from build123d import *

# Parameters (mm, degrees)
SKETCH1_R               = 32
BOSS_EXTRUDE1_DEPTH     = 15
SKETCH1_R_2             = 19
BOSS_EXTRUDE1_2_DEPTH   = 15
BOSS_EXTRUDE2_DEPTH     = 5
CUT_EXTRUDE1_DEPTH      = 84.026980949
CUT_EXTRUDE1_DEPTH_BACK = 84.026980949
SKETCH1_4_R             = 17
SKETCH1_4_R_2           = 10
BOSS_EXTRUDE3_START     = 15
SKETCH1_5_R             = 21.5
SKETCH1_5_R_2           = 17
BOSS_EXTRUDE3_DEPTH     = 15
CUT_EXTRUDE2_DEPTH      = 87.997008946
CUT_EXTRUDE2_DEPTH_BACK = 5
CUT_EXTRUDE2_START      = 15
SKETCH1_6_R             = 27.5
SKETCH1_6_R_2           = 21.5


with BuildPart() as part:
    # Sketch1 → Boss-Extrude1 (new, symmetric)
    with BuildSketch(Plane.XY):
        with Locations((-34.339012541, -15.619481103)):
            Circle(SKETCH1_R)
    extrude(amount=BOSS_EXTRUDE1_DEPTH, both=True)



with BuildPart() as body_2:
    # Sketch1 → Boss-Extrude1 2 (new, symmetric)
    with BuildSketch(Plane.XY):
        with Locations((36.527862472, 8.934256411)):
            Circle(SKETCH1_R_2)
    extrude(amount=BOSS_EXTRUDE1_2_DEPTH, both=True)


with BuildPart() as part_1:
    add(part.part)

    add(body_2.part)  # Boss-Extrude2 merges body 2
    # Sketch1<3> → Boss-Extrude2 (add, symmetric)
    with BuildSketch(Plane.XY):
        with BuildLine():
            ThreePointArc((-17.560856981, 11.629252739), (-6.402468571, -0.013408214), (-2.339012541, -15.619481103))
            ThreePointArc((-2.339012541, -15.619481103), (-2.421245933, -17.912115996), (-2.667523463, -20.192967692))
            ThreePointArc((-2.667523463, -20.192967692), (12.135506322, -12.174986093), (28.517182449, -8.294469763))
            ThreePointArc((28.517182449, -8.294469763), (17.876719368, 5.310051543), (22.64811714, 21.909335198))
            ThreePointArc((22.64811714, 21.909335198), (3.400059206, 13.419502104), (-17.560856981, 11.629252739))
        make_face()
    extrude(amount=BOSS_EXTRUDE2_DEPTH, both=True)

    # Sketch1<4> → Cut-Extrude1 (cut, two sides: drawn at the far end of the back side and taken through both)
    with BuildSketch(Plane.XY.offset(-CUT_EXTRUDE1_DEPTH_BACK)):
        with Locations((-34.339012541, -15.619481103)):
            Circle(SKETCH1_4_R)
        with Locations((36.527862472, 8.934256411)):
            Circle(SKETCH1_4_R_2)
    extrude(amount=CUT_EXTRUDE1_DEPTH + CUT_EXTRUDE1_DEPTH_BACK, mode=Mode.SUBTRACT)

    # Sketch1<5> → Boss-Extrude3 (add)
    with BuildSketch(Plane.XY.offset(BOSS_EXTRUDE3_START)):
        with Locations((-34.339012541, -15.619481103)):
            Circle(SKETCH1_5_R)
        with Locations((-34.339012541, -15.619481103)):
            Circle(SKETCH1_5_R_2, mode=Mode.SUBTRACT)
    extrude(amount=BOSS_EXTRUDE3_DEPTH)

    # Sketch1<6> → Cut-Extrude2 (cut, two sides: drawn at the far end of the back side and taken through both)
    with BuildSketch(Plane.XY.offset(CUT_EXTRUDE2_START - CUT_EXTRUDE2_DEPTH_BACK)):
        with Locations((-34.339012541, -15.619481103)):
            Circle(SKETCH1_6_R)
        with Locations((-34.339012541, -15.619481103)):
            Circle(SKETCH1_6_R_2, mode=Mode.SUBTRACT)
    extrude(amount=CUT_EXTRUDE2_DEPTH + CUT_EXTRUDE2_DEPTH_BACK, mode=Mode.SUBTRACT)


solid = part_1.part
Here's how the part is built. I have some questions about the finished solid (model axes, mm). A direction names the side the tool comes from. Round coordinates to 2 decimals unless told otherwise and drop trailing zeros. Write each loop counter-clockwise with the first axis right and the second up, starting at its lowest first coordinate (ties: lowest second). Pieces come first, ordered by that corner, then holes.
1. Suppose I cut it at C-C (y = 14). List the corners of the cut face in (x, z) for me, and give its area (3 significant figures).
2. Will these pins go through, and if not, where does the flat tip stop? pin 1 Ø1 at (y, z) = (-34.5, -1.5) entering from +X; pin 2 Ø1.5 at (y, z) = (19, 9) entering from +X; pin 3 Ø3 at (y, z) = (3.5, 2) entering from +X.
3. Suppose I cut it at B-B (y = -5.5). List the corners of the cut face in (x, z) for me, and give its area (3 significant figures).
4. Suppose I cut it at D-D (z = 13.5). List the corners of the cut face in (x, y) for me.
5. If we mould it in two halves opening along Y, with no side actions, what happens to faces 4 (the flat face through (45, 1, -15)), 5 (the cylindrical face through (-59.733, -35.091, 0.21)), 6 (the cylindrical face through (-14.478, -23.854, 19.86))? For each: released by +Y, released by -Y, zero draft, split by the parting line, or undercut.
6. Suppose I cut it at A-A (x = -39.5). List the corners of the cut face in (y, z) for me, and give its area (3 significant figures).
7. I need wall thicknesses on L1, parallel to X at y = -4.5, z = -7; L2, parallel to X at y = -13, z = 10.5; L3, parallel to Y at x = -35, z = 22. Which ranges of each line are inside material? Lowest first, please.
8. For faces 1 (the flat face through (-51, -30, 10)), 2 (the flat face through (45, 1, 15)), 3 (the cylindrical face through (54.65, 14.64, 0.21)), which set-ups out of +Z, -Z, +X, -X, +Y, -Y let a thin tool reach every point of the face, with its end or its side?
Answer sheet:
1. outline: (-46.45, -15) - (-22.23, -15) - (-22.23, 15) - (-46.45, 15) - close; (5.52, -5) - (18.22, -5) - (18.22, -15) - (27.91, -15) - (27.91, 15) - (18.22, 15) - (18.22, 5) - (5.52, 5) - close; (45.15, -15) - (54.84, -15) - (54.84, 15) - (45.15, 15) - close
1. area: 1,440 mm2
2. pin 1: stops at x = -8.14
2. pin 2: stops at x = 53.09
2. pin 3: stops at x = 55.12
3. outline: (-64.7, -15) - (-48, -15) - (-48, 30) - (-53.31, 30) - (-53.31, 10) - (-59.91, 10) - (-59.91, 15) - (-64.7, 15) - close; (-20.68, -15) - (-3.98, -15) - (-3.98, -5) - (24.17, -5) - (24.17, -15) - (48.88, -15) - (48.88, 15) - (24.17, 15) - (24.17, 5) - (-3.98, 5) - (-3.98, 15) - (-8.77, 15) - (-8.77, 10) - (-15.37, 10) - (-15.37, 30) - (-20.68, 30) - close
3. area: 2,120 mm2
4. outline: circle Ø64 at (-34.34, -15.62); circle Ø43 at (-34.34, -15.62); circle Ø38 at (36.53, 8.93); hole circle Ø55 at (-34.34, -15.62); hole circle Ø34 at (-34.34, -15.62); hole circle Ø20 at (36.53, 8.93)
5. face 4: zero draft
5. face 5: split by the parting line
5. face 6: undercut
6. outline: (-47.2, -15) - (-31.82, -15) - (-31.82, 30) - (-36.49, 30) - (-36.49, 10) - (-42.63, 10) - (-42.63, 15) - (-47.2, 15) - close; (0.58, -15) - (15.96, -15) - (15.96, 15) - (11.39, 15) - (11.39, 10) - (5.25, 10) - (5.25, 30) - (0.58, 30) - close
6. area: 1,000 mm2
7. L1: x = -64.34 to -47.2, -21.48 to -4.33, 23.09 to 49.96
7. L2: x = -66.23 to -61.71, -55.68 to -51.14, -17.54 to -13, -6.96 to -2.45
7. L3: y = -37.11 to -32.61, 1.37 to 5.87
8. face 1: +Z
8. face 2: +Z, +X, +Y, -Y
8. face 3: none
